Could you check a few things on this model? Use its own coordinates, in mm. Round coordinates to 2 decimals unless told otherwise and drop trailing zeros. Loops run counter-clockwise (first coordinate to the right, second up) from the corner with the lowest first, then second, coordinate; pieces in that order, holes last. Notation, with made-up numbers: (82, 30.5) -> (90, 30.5) arc R17 ccw to (90, 49.5) -> close; hole circle Ø9 at (71.25, 69). An arc over 180 degrees is marked (long way). Write each question's results on one line, items separated by ' | '.
from build123d import *

# Parameters (mm, degrees)
SKETCH1_R               = 90
BOSS_EXTRUDE1_DEPTH     = 3
CUT_EXTRUDE1_DEPTH      = 1
CUT_EXTRUDE1_DEPTH_BACK = 3
CUT_EXTRUDE2_DEPTH      = 1
CUT_EXTRUDE2_DEPTH_BACK = 3
SKETCH5_W               = 3
SKETCH5_H               = 14
CUT_EXTRUDE4_DEPTH      = 3
SKETCH6_W               = 3
SKETCH6_H               = 14
CUT_EXTRUDE5_DEPTH      = 3
SKETCH8_W               = 3
SKETCH8_H               = 14
CUT_EXTRUDE7_DEPTH      = 3
SKETCH9_W               = 14
SKETCH9_H               = 3
CUT_EXTRUDE8_DEPTH      = 3
SKETCH10_W              = 14
SKETCH10_H              = 3
CUT_EXTRUDE9_DEPTH      = 3
SKETCH11_W              = 14
SKETCH11_H              = 3
CUT_EXTRUDE10_DEPTH     = 3
SKETCH12_W              = 14
SKETCH12_H              = 3
CUT_EXTRUDE11_DEPTH     = 3
SKETCH13_W              = 14
SKETCH13_H              = 3
CUT_EXTRUDE12_DEPTH     = 3
SKETCH14_W              = 14
SKETCH14_H              = 3
CUT_EXTRUDE13_DEPTH     = 3
SKETCH15_R              = 7
CUT_EXTRUDE14_DEPTH     = 3


with BuildPart() as part:
    # Sketch1 → Boss-Extrude1 (new body)
    with BuildSketch(Plane(origin=(0, 0, 0), x_dir=(1, 0, 0), z_dir=(0, 1, 0))):
        Circle(SKETCH1_R)
    extrude(amount=BOSS_EXTRUDE1_DEPTH)

    # Sketch2 → Cut-Extrude1 (cut, two sides)
    with BuildSketch(Plane(origin=(0, 3, 0), x_dir=(1, 0, 0), z_dir=(0, 1, 0))) as cut_extrude1_sk:
        Polygon((-52.5, -516.266848974), (-52.5, -73.100957586), (-52.5, -43), (-79.063265807, -43), (-522.229157195, -43), (-1151.30715458, -667.375610001), (-681.577997385, -1140.642458975), align=None)
    extrude(amount=CUT_EXTRUDE1_DEPTH, mode=Mode.SUBTRACT)
    extrude(cut_extrude1_sk.sketch, amount=-CUT_EXTRUDE1_DEPTH_BACK, mode=Mode.SUBTRACT)

    # Sketch3 → Cut-Extrude2 (cut, two sides)
    with BuildSketch(Plane(origin=(0, 3, 0), x_dir=(1, 0, 0), z_dir=(0, 1, 0))) as cut_extrude2_sk:
        Polygon((52.5, -516.266848974), (52.5, -73.100957586), (52.5, -43), (79.063265807, -43), (522.229157195, -43), (1151.30715458, -667.375610001), (681.577997385, -1140.642458975), align=None)
    extrude(amount=CUT_EXTRUDE2_DEPTH, mode=Mode.SUBTRACT)
    extrude(cut_extrude2_sk.sketch, amount=-CUT_EXTRUDE2_DEPTH_BACK, mode=Mode.SUBTRACT)

    # Sketch5 → Cut-Extrude4 (cut)
    with BuildSketch(Plane(origin=(0, 3, 0), x_dir=(1, 0, 0), z_dir=(0, 1, 0))):
        with Locations((0, 25)):
            Rectangle(SKETCH5_W, SKETCH5_H)
    extrude(amount=-CUT_EXTRUDE4_DEPTH, mode=Mode.SUBTRACT)

    # Sketch6 → Cut-Extrude5 (cut)
    with BuildSketch(Plane(origin=(0, 3, 0), x_dir=(1, 0, 0), z_dir=(0, 1, 0))):
        with Locations((0, 65)):
            Rectangle(SKETCH6_W, SKETCH6_H)
    extrude(amount=-CUT_EXTRUDE5_DEPTH, mode=Mode.SUBTRACT)

    # Sketch8 → Cut-Extrude7 (cut)
    with BuildSketch(Plane(origin=(0, 3, 0), x_dir=(1, 0, 0), z_dir=(0, 1, 0))):
        with Locations((0, -65)):
            Rectangle(SKETCH8_W, SKETCH8_H)
    extrude(amount=-CUT_EXTRUDE7_DEPTH, mode=Mode.SUBTRACT)

    # Sketch9 → Cut-Extrude8 (cut)
    with BuildSketch(Plane(origin=(0, 3, 0), x_dir=(1, 0, 0), z_dir=(0, 1, 0))):
        with Locations((-25, 0)):
            Rectangle(SKETCH9_W, SKETCH9_H)
    extrude(amount=-CUT_EXTRUDE8_DEPTH, mode=Mode.SUBTRACT)

    # Sketch10 → Cut-Extrude9 (cut)
    with BuildSketch(Plane(origin=(0, 3, 0), x_dir=(1, 0, 0), z_dir=(0, 1, 0))):
        with Locations((-65, 0)):
            Rectangle(SKETCH10_W, SKETCH10_H)
    extrude(amount=-CUT_EXTRUDE9_DEPTH, mode=Mode.SUBTRACT)

    # Sketch11 → Cut-Extrude10 (cut)
    with BuildSketch(Plane(origin=(0, 3, 0), x_dir=(1, 0, 0), z_dir=(0, 1, 0))):
        with Locations((25, 0)):
            Rectangle(SKETCH11_W, SKETCH11_H)
    extrude(amount=-CUT_EXTRUDE10_DEPTH, mode=Mode.SUBTRACT)

    # Sketch12 → Cut-Extrude11 (cut)
    with BuildSketch(Plane(origin=(0, 3, 0), x_dir=(1, 0, 0), z_dir=(0, 1, 0))):
        with Locations((65, 0)):
            Rectangle(SKETCH12_W, SKETCH12_H)
    extrude(amount=-CUT_EXTRUDE11_DEPTH, mode=Mode.SUBTRACT)

    # Sketch13 → Cut-Extrude12 (cut)
    with BuildSketch(Plane(origin=(0, 3, 0), x_dir=(1, 0, 0), z_dir=(0, 1, 0))):
        with Locations((-39, 45)):
            Rectangle(SKETCH13_W, SKETCH13_H)
    extrude(amount=-CUT_EXTRUDE12_DEPTH, mode=Mode.SUBTRACT)

    # Sketch14 → Cut-Extrude13 (cut)
    with BuildSketch(Plane(origin=(0, 3, 0), x_dir=(1, 0, 0), z_dir=(0, 1, 0))):
        with Locations((39, 45)):
            Rectangle(SKETCH14_W, SKETCH14_H)
    extrude(amount=-CUT_EXTRUDE13_DEPTH, mode=Mode.SUBTRACT)

    # Sketch15 → Cut-Extrude14 (cut)
    with BuildSketch(Plane(origin=(0, 3, 0), x_dir=(1, 0, 0), z_dir=(0, 1, 0))):
        with Locations((-15, 23.5)):
            Circle(SKETCH15_R)
        with Locations((15, 23.5)):
            Circle(SKETCH15_R)
    extrude(amount=-CUT_EXTRUDE14_DEPTH, mode=Mode.SUBTRACT)


solid = part.part
1) I want a section at B-B, the plane z = -23.5. Write out the boundary of the cut face in (x, y).
Model answer:
outline: (-86.88, 0) -> (-22, 0) -> (-22, 3) -> (-86.88, 3) -> close; (-8, 0) -> (-1.5, 0) -> (-1.5, 3) -> (-8, 3) -> close; (1.5, 0) -> (8, 0) -> (8, 3) -> (1.5, 3) -> close; (22, 0) -> (86.88, 0) -> (86.88, 3) -> (22, 3) -> close
2) If we mould it in two halves opening along X, with no side actions, what happens to faces 1 (the cylindrical face through (2.606, 1.479, -89.962)), 2 (the cylindrical face through (-20.555, 1.521, -19.241)), 3 (the flat face through (-1, 3, -1))? For each: released by +X, released by -X, zero draft, split by the parting line, or undercut.
Model answer:
face 1: split by the parting line | face 2: undercut | face 3: zero draft
3) I want a section at D-D, the plane y = 1.3. Give the number of separate pieces and of enclosed holes in the cut face, plus the area to 3 significant figures.
Model answer:
separate pieces: 1 | enclosed holes: 11 | area: 23,800 mm2
4) I want a section at C-C, the plane z = -64. Write out the boundary of the cut face in (x, y).
Model answer:
outline: (-63.28, 0) -> (-1.5, 0) -> (-1.5, 3) -> (-63.28, 3) -> close; (1.5, 0) -> (63.28, 0) -> (63.28, 3) -> (1.5, 3) -> close
5) I need wall thicknesses on line 1 (Z direction, x = -1, y = 1.4); line 2 (X direction, y = 1.3, z = -23.5); line 3 (X direction, y = 0.55, z = -25.5). Which ranges of each line are inside material? Lowest first, please.
Model answer:
line 1: z = -89.99 to -72, -58 to -32, -18 to 58, 72 to 89.99 | line 2: x = -86.88 to -22, -8 to -1.5, 1.5 to 8, 22 to 86.88 | line 3: x = -86.31 to -21.71, -8.29 to -1.5, 1.5 to 8.29, 21.71 to 86.31
6) I want a section at A-A, the plane x = 15. Write out the boundary of the cut face in (y, z), plus the area to 3 significant figures.
Model answer:
outline: (0, -88.74) -> (3, -88.74) -> (3, -30.5) -> (0, -30.5) -> close; (0, -16.5) -> (3, -16.5) -> (3, 88.74) -> (0, 88.74) -> close | area: 490 mm2
7) I'm going to push flat-ended pins straight in: pin 1 (2 mm diameter, centred on x = 67, z = 10.5, fed in from -Y); pin 2 (1.5 mm diameter, centred on y = 2.5, z = -25, fed in from -X); pin 3 (1.5 mm diameter, centred on x = 27, y = 1.5, fed in from +Z); pin 4 (0.9 mm diameter, centred on y = 2, z = -45.5, fed in from -X). Where does each tip first touch, or does it pass through?
Model answer:
pin 1: stops at y = 0 | pin 2: stops at x = -86.67 | pin 3: stops at z = 86.09 | pin 4: stops at x = -77.91
